Autodesk Fusion 360 part; units mm, degrees
sketch "Esquisse1" plane through (0, 0, 0) normal (1, 0, 0) x (0, 0, -1)
  circle A0 centre (0, 0) radius 10 construction
  circle A1 centre (0, 0) radius 15 construction
  line L0 (15, -35) -> (15, 0) construction
  line L1 (-15, -35) -> (-15, 0) construction
  line L2 (4, 1) -> (25, 1) construction
  line L3 (4, -1) -> (25, -1) construction
  line L4 (25, -1) -> (25, -7) construction
  line L5 (25, -7) -> (13.2665, -7) construction
  line L6 (25, 1) -> (25, 7) construction
  line L7 (25, 7) -> (13.2665, 7) construction
  line L8 (-15, -35) -> (-55, -35) construction
  line L9 (-55, -35) -> (-55, -45) construction
  line L10 (15, -35) -> (55, -35) construction
  line L11 (55, -35) -> (55, -45) construction
  line L12 (55, -45) -> (-55, -45) construction
  line L13 (55, -45) -> (-55, -45)
  line L14 (-55, -45) -> (-55, -35)
  line L15 (-55, -35) -> (-15, -35)
  line L16 (-15, -35) -> (-15, 0)
  line L17 (13.2665, 7) -> (25, 7)
  line L18 (25, 7) -> (25, 1)
  line L19 (25, 1) -> (9.9499, 1)
  line L20 (9.9499, -1) -> (25, -1)
  line L21 (25, -1) -> (25, -7)
  line L22 (25, -7) -> (15, -7)
  line L23 (15, -7) -> (15, -35)
  line L24 (15, -35) -> (55, -35)
  line L25 (55, -35) -> (55, -45)
  arc A2 (13.2665, 7) -> (-15, 0) centre (0, 0) ccw
  arc A3 (9.9499, 1) -> (9.9499, -1) centre (0, 0) ccw
  dimension "d58" = 20
  dimension "d59" = 30
  dimension "d60" = 10
  dimension "d61" = 10
  dimension "d62" = 45
  dimension "d63" = 10
  dimension "d64" = 10
extrude "Extrusion8" add sketch "Esquisse1" along normal blind 15
fillet "Congé9" radius 7.5 4 edges at (15, -40, -55) (0, -40, -55) (15, -40, 55) (0, -40, 55)
fillet "Congé10" radius 5 2 edges at (7.5, -35, -15) (7.5, -35, 15)
sketch "Esquisse8" plane through (0, -35, 0) normal (0, 1, 0) x (-1, 0, 0)
  line L0 (-15, 20) -> (0, 20)
  line L1 (0, 20) -> (0, 47.5)
  arc A0 (0, 47.5) -> (-15, 47.5) centre (-7.5, 47.5) ccw
  line L2 (-15, 47.5) -> (-15, 20)
  line L3 (0, 47.5) -> (-15, 47.5) construction
  line L4 (-7.5, 55) -> (-7.5, 20) construction
  line L5 (0, 27.5) -> (-15, 27.5) construction
  line L6 (-2.5, 47.5) -> (-2.5, 27.5)
  line L7 (-5.5, 47.5) -> (-5.5, 27.5)
  arc A1 (-5.5, 47.5) -> (-7.5, 49.5) centre (-7.5, 47.5) ccw
  arc A2 (-2.5, 47.5) -> (-7.5, 52.5) centre (-7.5, 47.5) ccw
  arc A3 (-7.5, 25.5) -> (-5.5, 27.5) centre (-7.5, 27.5) ccw
  arc A4 (-7.5, 22.5) -> (-2.5, 27.5) centre (-7.5, 27.5) ccw
  arc A5 (-12.5, 27.5) -> (-7.5, 22.5) centre (-7.5, 27.5) ccw
  arc A6 (-9.5, 27.5) -> (-7.5, 25.5) centre (-7.5, 27.5) ccw
  line L8 (-9.5, 47.5) -> (-9.5, 27.5)
  line L9 (-12.5, 47.5) -> (-12.5, 27.5)
  arc A7 (-7.5, 52.5) -> (-12.5, 47.5) centre (-7.5, 47.5) ccw
  arc A8 (-7.5, 49.5) -> (-9.5, 47.5) centre (-7.5, 47.5) ccw
  line L10 (10, 0) -> (-30, 0)
  line L11 (-12.5, -47.5) -> (-12.5, -27.5)
  line L12 (-2.5, -47.5) -> (-2.5, -27.5)
  arc A9 (-7.5, -49.5) -> (-5.5, -47.5) centre (-7.5, -47.5) ccw
  arc A10 (-7.5, -52.5) -> (-2.5, -47.5) centre (-7.5, -47.5) ccw
  line L13 (-5.5, -47.5) -> (-5.5, -27.5)
  line L14 (0, -27.5) -> (-15, -27.5) construction
  arc A11 (-2.5, -27.5) -> (-7.5, -22.5) centre (-7.5, -27.5) ccw
  arc A12 (-5.5, -27.5) -> (-7.5, -25.5) centre (-7.5, -27.5) ccw
  arc A13 (-9.5, -47.5) -> (-7.5, -49.5) centre (-7.5, -47.5) ccw
  arc A14 (-12.5, -47.5) -> (-7.5, -52.5) centre (-7.5, -47.5) ccw
  line L15 (0, -47.5) -> (-15, -47.5) construction
  arc A15 (-7.5, -22.5) -> (-12.5, -27.5) centre (-7.5, -27.5) ccw
  line L16 (-9.5, -47.5) -> (-9.5, -27.5)
  arc A16 (-7.5, -25.5) -> (-9.5, -27.5) centre (-7.5, -27.5) ccw
  point P0 (-15, -47.5)
  point P1 (-7.5, -47.5)
  point P2 (0, -47.5)
  dimension "d71" = 20
  dimension "d72" = 5
  dimension "d73" = 2
extrude "Extrusion9" cut sketch "Esquisse8" against normal blind 20 contours L7 A1 A3 A6 L8 A8 | A9 L13 A12 A13 L16 A16
extrude "Extrusion10" cut sketch "Esquisse8" against normal blind 4 contours L6 A2 A4 A5 L9 A7 | L11 L12 A10 A11 A14 A15
sketch "Esquisse9" plane through (0, -7, 0) normal (0, -1, 0) x (1, 0, 0)
  line L0 (0, -15) -> (0, -25)
  line L1 (0, -25) -> (15, -25)
  line L2 (15, -25) -> (15, -15)
  line L3 (15, -15) -> (0, -15)
  line L4 (15, -25) -> (0, -15) construction
  line L5 (15, -15) -> (0, -25) construction
  circle A0 centre (7.5, -20) radius 2
  dimension "d78" = 4
extrude "Extrusion11" cut sketch "Esquisse9" against normal blind 35 contours A0
fillet "Congé11" radius 10 1 edges at (7.5, 7, -13.2665)
ref_plane "Plan de construction2" through (7.5, 12, -19.1332) normal (0, 1, 0) x (0, 0, 1)
sketch "Esquisse10" plane through (7.5, 12, -21.6652) normal (0, 1, 0) x (1, 0, 0)
  arc A0 (1.101, -3.3348) -> (-1.101, -3.3348) centre (0, -1.6652) ccw
  circle A1 centre (0, -1.6652) radius 5
  dimension "d84" = 10
extrude "Extrusion12" cut sketch "Esquisse10" against normal up to surface (5 mm away)
fillet "Congé12" radius 5 4 edges at (15, -4, -25) (15, 4, -25) (0, 4, -25) (0, -4, -25)
fillet "Congé13" radius 1 23 edges at (0, -15, 15) (0, -33.5355, 16.4645) (0, -35, 33.75) (7.5, -35, 55) (15, -35, 33.75) (15, -33.5355, 16.4645) (15, -15, 15) (15, 13.9638, 5.4785) (15, 7.8348, -14.3303) (15, 7, -19.1652) (13.5355, 7, -23.5355) (7.5, 7, -25) (1.4645, 7, -23.5355) (0, 7, -19.1652) (0, 7.8348, -14.3303) (0, 13.9638, 5.4785) (0, -18.5, -15) (0, -33.5355, -16.4645) (0, -35, -33.75) (7.5, -35, -55) (15, -35, -33.75) (15, -33.5355, -16.4645) (15, -18.5, -15)
Geometry: final body of the model. Coordinates: model frame, mm. A direction names the side the tool comes from. Coordinates: 2 decimals unless noted, no trailing zeros. Loops run counter-clockwise (first coordinate to the right, second up) from the corner with the lowest first, then second, coordinate; pieces in that order, holes last. Notation, with made-up numbers: (47.25, 0.25) -> (59.25, 0.25) arc R15 cw to (59.25, 28.25) -> close; hole circle Ø4 at (-12, -31). An arc over 180 degrees is marked (long way). Use a Markdown table: item, result. Add a question column.
(1) Pin query (flat end, axial travel): pin 1 Ø4 at (x, z) = (7.5, -11.5) entering from +Y; pin 2 Ø4.5 at (x, z) = (9.5, -17) entering from +Y; pin 3 Ø2.5 at (x, z) = (9.5, -21.5) entering from +Y; pin 4 Ø16 at (y, z) = (0, 0) entering from +X. Return the tip coordinate at first contact, or that it passes through.
(2) Section query B-B, the plane y = -28. Return loops of the section in (x, z), plus the area to 3 significant figures.
(3) Section query A-A, the plane z = 0. Return loops of the section in (x, y), plus the area to 3 significant figures.
(4) Mould query, pull axis X, two halves, no side actions, for faces 5 (the cylindrical face through (7.5, -42, -49.5)), 6 (the flat face through (7, -15, 15)), 7 (the cylindrical face through (2.138, -40.437, 52.745)). Classes: pulls with the +X half, pulls with the -X half, needs draft (parallel to the pull), parting line crosses it, or undercut.
(5) Line query: line 1 along Y through (x, z) = (10.5, -24.5); line 2 along X through (y, z) = (-41, 37); line 3 along Y through (x, z) = (3.25, 0). Output: solid intervals per line, ascending.
(6) Access query for faces 1 (the flat face through (9, 7, -18)), 2 (the flat face through (9.5, -42, 38)), 3 (the cylindrical face through (13, 3, -24)), 4 (the flat face through (2, -35, 35)). Directions: +Z, -Z, +X, -X, +Y, -Y. A direction counts if a zero-diameter tool reaches every point of the face in a straight line with its end or side. Return the directions, or none.
(7) Section query C-C, the plane z = 34. Return loops of the section in (x, y), plus the area to 3 significant figures.
Answer:
| question | item | result |
|---|---|---|
| 1 | pin 1 | stops at y = 11.61 |
| 1 | pin 2 | stops at y = 7.66 |
| 1 | pin 3 | stops at y = 7 |
| 1 | pin 4 | passes through |
| 2 | outline | (0, -14) arc R1 ccw to (1, -15) -> (14, -15) arc R1 ccw to (15, -14) -> (15, 14) arc R1 ccw to (14, 15) -> (1, 15) arc R1 ccw to (0, 14) -> close |
| 2 | area | 449 mm^2 |
| 3 | outline | (0, -45) -> (15, -45) -> (15, -10) -> (0, -10) -> close; (0, 10) -> (15, 10) -> (15, 14) arc R1 ccw to (14, 15) -> (1, 15) arc R1 ccw to (0, 14) -> close |
| 3 | area | 600 mm^2 |
| 4 | face 5 | undercut |
| 4 | face 6 | needs draft |
| 4 | face 7 | pulls with the -X half |
| 5 | line 1 | y = -45 to -39, -7 to -1, 1 to 6.85 |
| 5 | line 2 | x = 0 to 5.5, 9.5 to 15 |
| 5 | line 3 | y = -45 to -10, 10 to 15 |
| 6 | face 1 | -Z, +Y |
| 6 | face 2 | +Y, -Y |
| 6 | face 3 | -Z, +X, +Y |
| 6 | face 4 | +Z, +X, -X, +Y |
| 7 | outline | (0, -45) -> (5.5, -45) -> (5.5, -39) -> (2.5, -39) -> (2.5, -35) -> (1, -35) arc R1 ccw to (0, -36) -> close; (9.5, -45) -> (15, -45) -> (15, -36) arc R1 ccw to (14, -35) -> (12.5, -35) -> (12.5, -39) -> (9.5, -39) -> close |
| 7 | area | 85.6 mm^2 |
